For this review, take the finished solid that the model builds, in its own axes (mm). Give positions to 0.01 mm unless a question says otherwise; leave off trailing zeros. Loops run counter-clockwise (first coordinate to the right, second up) from the corner with the lowest first, then second, coordinate; pieces in that order, holes last. Notation, with made-up numbers: (57, 10.25) - (110, 10.25) arc R25 cw to (110, 22.25) - close; hole circle Ø3 at (43, 1). An arc over 180 degrees is marked (long way). Put each result on its own line as item: value. Start each with the question number.
from build123d import *

# Parameters (mm, degrees)
SKETCH_1_W      = 100
SKETCH_1_H      = 32
SKETCH_1_R      = 2
SKETCH_1_R_2    = 1.5
SKETCH_1_W_2    = 40.8
SKETCH_1_H_2    = 20.8
EXTRUDE_1_DEPTH = 3
FILLET_1_R      = 0.5
FILLET_2_R      = 2


with BuildPart() as part:
    # 草图1 → 凸台-拉伸1 (new body)
    with BuildSketch(Plane(origin=(0, 0, 0), x_dir=(1, 0, 0), z_dir=(0, 1, 0))):
        Rectangle(SKETCH_1_W, SKETCH_1_H)
        with Locations(Location((24.75, 5, 0), (0, 0, 270))):
            Circle(SKETCH_1_R, mode=Mode.SUBTRACT)
        with Locations(Location((24.75, -5, 0), (0, 0, 90))):
            Circle(SKETCH_1_R, mode=Mode.SUBTRACT)
        with Locations(Location((-24.75, -5, 0), (0, 0, 270))):
            Circle(SKETCH_1_R, mode=Mode.SUBTRACT)
        with Locations(Location((-24.75, 5, 0), (0, 0, 90))):
            Circle(SKETCH_1_R, mode=Mode.SUBTRACT)
        with Locations(Location((-44, 8, 0), (0, 0, 270))):
            Circle(SKETCH_1_R_2, mode=Mode.SUBTRACT)
        with Locations(Location((44, 8, 0), (0, 0, 90))):
            Circle(SKETCH_1_R_2, mode=Mode.SUBTRACT)
        with Locations(Location((44, -8, 0), (0, 0, 270))):
            Circle(SKETCH_1_R_2, mode=Mode.SUBTRACT)
        with Locations(Location((-44, -8, 0), (0, 0, 90))):
            Circle(SKETCH_1_R_2, mode=Mode.SUBTRACT)
        Rectangle(SKETCH_1_W_2, SKETCH_1_H_2, mode=Mode.SUBTRACT)
    extrude(amount=EXTRUDE_1_DEPTH)

    # 圆角1
    fillet_1_edges = [part.edges().sort_by_distance(p)[0] for p in [
        (20.4, 1.5, 10.4),
        (20.4, 1.5, -10.4),
        (-20.4, 1.5, -10.4),
        (-20.4, 1.5, 10.4),
    ]]
    fillet(fillet_1_edges, radius=FILLET_1_R)

    # 圆角2
    fillet_2_edges = [part.edges().sort_by_distance(p)[0] for p in [
        (50, 1.5, 16),
        (-50, 1.5, 16),
        (-50, 1.5, -16),
        (50, 1.5, -16),
    ]]
    fillet(fillet_2_edges, radius=FILLET_2_R)


solid = part.part
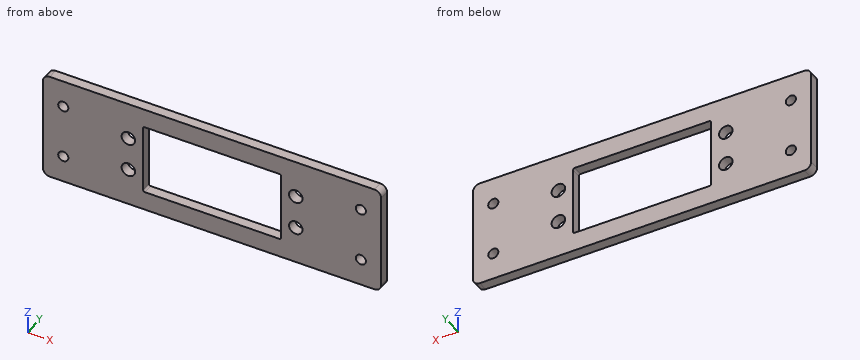
1) Take a section at C-C on x = 44. State the section outline as (y, z) points, and give its area (3 significant figures).
2) Insertion check: P1, Ø4, axis at x = -44, z = 8, coming from the +Y side; P2, Ø3, axis at x = -24.75, z = 5, coming from the -Y side. Each pin has a flat end and moves straight along its axis. Give the tip position at first contact, or say it passes through.
3) Wall thickness on probe 1 along X at (y, z) = (0.65, -8); probe 2 along Z at (x, y) = (8, 2.8); probe 3 along X at (y, z) = (1.7, -7.5): over which ranges is each line inside the solid? List them lowest first.
4) Take a section at D-D on y = 2.5. State how many separate pieces and enclosed holes the cut face has, and give its area (3 significant figures).
5) Take a section at A-A on z = 5. State the section outline as (x, y) points, and give its area (3 significant figures).
6) Take a section at B-B on x = 2.5. State the section outline as (y, z) points.
Answers follow:
1. outline: (0, -16) - (3, -16) - (3, -9.5) - (0, -9.5) - close; (0, -6.5) - (3, -6.5) - (3, 6.5) - (0, 6.5) - close; (0, 9.5) - (3, 9.5) - (3, 16) - (0, 16) - close
1. area: 78.0 mm2
2. P1: y = 3
2. P2: through
3. probe 1: -50 to -45.5, -42.5 to -20.4, 20.4 to 42.5, 45.5 to 50
3. probe 2: -16 to -10.4, 10.4 to 16
3. probe 3: -50 to -45.41, -42.59 to -20.4, 20.4 to 42.59, 45.41 to 50
4. separate pieces: 1
4. enclosed holes: 9
4. area: 2,270 mm2
5. outline: (-50, 0) - (-26.75, 0) - (-26.75, 3) - (-50, 3) - close; (-22.75, 0) - (-20.4, 0) - (-20.4, 3) - (-22.75, 3) - close; (20.4, 0) - (22.75, 0) - (22.75, 3) - (20.4, 3) - close; (26.75, 0) - (50, 0) - (50, 3) - (26.75, 3) - close
5. area: 154 mm2
6. outline: (0, -16) - (3, -16) - (3, -10.4) - (0, -10.4) - close; (0, 10.4) - (3, 10.4) - (3, 16) - (0, 16) - close
